```python
from build123d import *

# Parameters (mm, degrees)
F0_W     = 50.8
F0_H     = 203.2
F1_DEPTH = 63.5
F2_W     = 25.4
F2_H     = 6.35
F5_DEPTH = 6.35
F6_R     = 5.08


with BuildPart() as f1:
    # F0 (on Front) → F1 (new body, symmetric)
    with BuildSketch(Plane.XZ):
        with Locations((-228.6, 0)):
            Rectangle(F0_W, F0_H)
        Polygon((-203.2, 101.6), (203.2, 101.6), (254, 101.6), (254, 152.4), (-254, 152.4), (-254, 101.6), align=None)
        with Locations((228.6, 0)):
            Rectangle(F0_W, F0_H)
    extrude(amount=F1_DEPTH, both=True)

    # F2 (on Front) → F3 (revolve, cut)
    with BuildSketch(Plane.XZ):
        with Locations((215.9, 98.425)):
            Rectangle(F2_W, F2_H)
        with Locations((-215.9, 98.425)):
            Rectangle(F2_W, F2_H)
    revolve(axis=Axis((-215.9, 0, 95.25), (1, 0, 0)), mode=Mode.SUBTRACT)

    # F4 (on Front) → F5 (cut, symmetric)
    with BuildSketch(Plane.XZ):
        Polygon((203.2, 83.82), (203.2, 0), (203.2, -99.06), (228.6, -99.06), (228.6, -92.71), (228.6, 83.82), align=None)
        Polygon((-203.2, -99.06), (-203.2, 0), (-203.2, 83.82), (-228.6, 83.82), (-228.6, -99.06), align=None)
    extrude(amount=F5_DEPTH, both=True, mode=Mode.SUBTRACT)

    # F6
    f6_edges = [f1.edges().sort_by_distance(p)[0] for p in [
        (-215.9, -6.35, 83.82),
        (-215.9, 6.35, 83.82),
        (-215.9, 6.35, -99.06),
        (-215.9, -6.35, -99.06),
        (215.9, -6.35, 83.82),
        (215.9, 6.35, 83.82),
        (215.9, -6.35, -99.06),
        (215.9, 6.35, -99.06),
    ]]
    fillet(f6_edges, radius=F6_R)


solid = f1.part
```
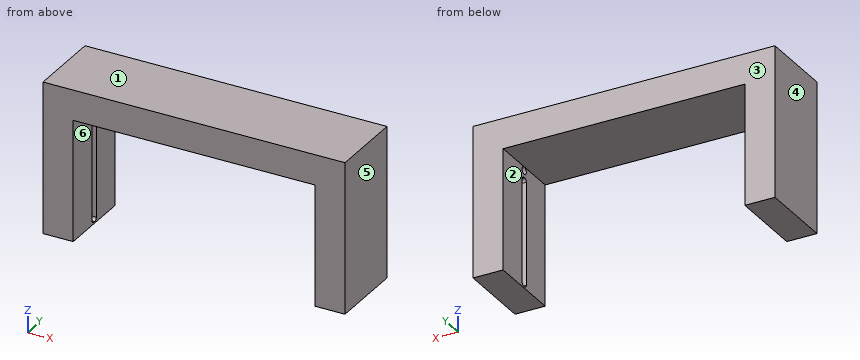
Build history of the part. All positions in model axes, mm. Face numbers are marked on the shaded views. A direction names the side the tool comes from. Coordinates: 2 decimals unless noted, no trailing zeros. Order: outer loops, then holes, each group sorted by start corner. A loop starts at its lowest first (then second) coordinate and runs counter-clockwise, first axis right, second up.
Item 1: Saw through at B-B on y = 42. List the corners of the cut face in (x, z).
Filled in:
outline: (-254, -101.6) - (-203.2, -101.6) - (-203.2, 101.6) - (203.2, 101.6) - (203.2, -101.6) - (254, -101.6) - (254, 152.4) - (-254, 152.4) - close
Item 2: Tool access for the marked faces 1 and 2: list every direction of +Z, -Z, +X, -X, +Y, -Y with a clear straight run to the whole face (end or side of a thin tool).
Filled in:
face 1: +Z, +X, -X, +Y, -Y
face 2: -Z, +Y, -Y
Item 3: Drop a flat-ended pin along its axis: pin 1 Ø2 at (x, y) = (-56, 31.5) entering from -Z. Give the stop position or say it passes through.
Filled in:
pin 1: stops at z = 101.6
Item 4: Drill centre lines: L1, parallel to Z at x = 222.5, y = 0; L2, parallel to X at y = 35.5, z = 12; L3, parallel to Y at x = 213, z = 95. Where is each one in solid material? Low to high.
Filled in:
L1: z = -101.6 to -99.06, 83.82 to 88.9, 101.6 to 152.4
L2: x = -254 to -203.2, 203.2 to 254
L3: y = -63.5 to -6.35, 6.35 to 63.5
Item 5: Mould opens along X. For the marked faces 3, 4, 5 and 6 say: released by +X, released by -X, zero draft, split by the parting line, or undercut.
Filled in:
face 3: zero draft
face 4: released by -X
face 5: released by +X
face 6: undercut
Item 6: Saw through at A-A on z = 95.25. List the corners of the cut face in (x, y), then the cut area to 3 significant figures.
Filled in:
outline: (-254, -63.5) - (-203.2, -63.5) - (-203.2, -6.35) - (-228.6, -6.35) - (-228.6, 6.35) - (-203.2, 6.35) - (-203.2, 63.5) - (-254, 63.5) - close; (203.2, -63.5) - (254, -63.5) - (254, 63.5) - (203.2, 63.5) - (203.2, 6.35) - (228.6, 6.35) - (228.6, -6.35) - (203.2, -6.35) - close
area: 12,300 mm2
Item 7: Saw through at C-C on x = 109. List the corners of the cut face in (y, z), then the cut area to 3 significant figures.
Filled in:
outline: (-63.5, 101.6) - (63.5, 101.6) - (63.5, 152.4) - (-63.5, 152.4) - close
area: 6,450 mm2
